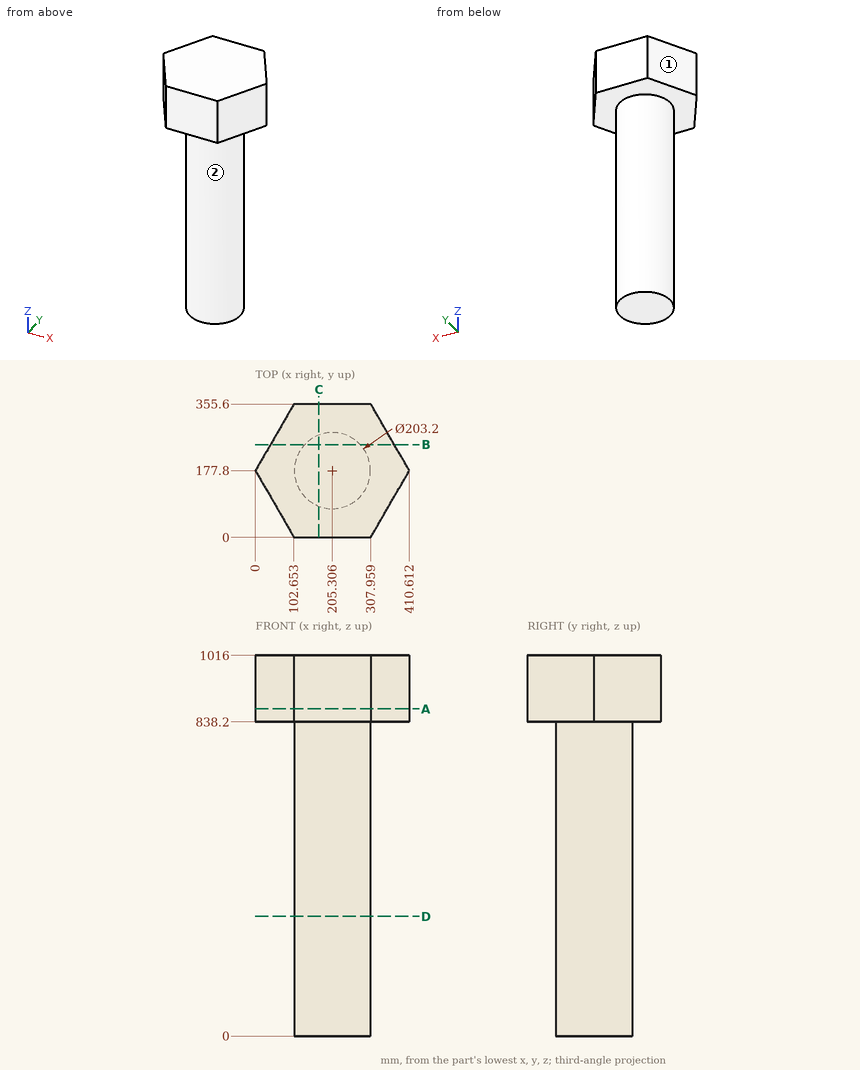
Drawing for the job (mm, zero at the part's lowest x, y, z). A direction names the side the tool comes from. Give positions to 0.01 mm unless a question says otherwise; leave off trailing zeros. Order: outer loops, then holes, each group sorted by start corner. A loop starts at its lowest first (then second) coordinate and runs counter-clockwise, first axis right, second up. Notation, with made-up numbers: (30, -30.75) -> (42, -30.75) arc R30 ccw to (42, 5.25) -> close; hole circle Ø10 at (69.5, 70.25). An arc over 180 degrees is marked (long way). Use one line per item in the form item = value.
(1) Saw through at A-A (z = 873). Write the cut outline in (x, y).
Solution:
outline = (0, 177.8) -> (102.65, 0) -> (307.96, 0) -> (410.61, 177.8) -> (307.96, 355.6) -> (102.65, 355.6) -> close
(2) Flat gauge pins, fed straight in: P1, Ø5, axis at x = 135.5, z = 650, coming from the +Y side; P2, Ø2, axis at y = 155, z = 817.5, coming from the -X side; P3, Ø5, axis at x = 112, y = 270.5, coming from the -Z side. Where does each tip first touch, or does it go through?
Solution:
P1 = 253.91
P2 = 106.07
P3 = 838.2
(3) Saw through at D-D (z = 319.5). Write the cut outline in (x, y) (1 decimal).
Solution:
outline = circle Ø203.2 at (205.3, 177.8)
(4) Saw through at C-C (x = 169.5). Write the cut outline in (y, z), then the cut area to 3 significant figures.
Solution:
outline = (0, 838.2) -> (82.72, 838.2) -> (82.72, 0) -> (272.88, 0) -> (272.88, 838.2) -> (355.6, 838.2) -> (355.6, 1016) -> (0, 1016) -> close
area = 223,000 mm²
(5) Drill centre lines: line 1 (Z direction, x = 294, y = 87); line 2 (X direction, y = 177, z = 565); line 3 (Y direction, x = 204.5, z = 168.5). Where is each one in solid material? Low to high. Write a range as from..to.
Solution:
line_1 = 838.2..1016
line_2 = 103.71..306.9
line_3 = 76.2..279.4
(6) Tool access for the marked faces 1 and 2: list every direction of +Z, -Z, +X, -X, +Y, -Y with a clear straight run to the whole face (end or side of a thin tool).
Solution:
face_1 = +Z, -Z, -X, +Y
face_2 = -Z
(7) Saw through at B-B (y = 247.5). Write the cut outline in (x, z), then the cut area to 3 significant figures.
Solution:
outline = (40.24, 838.2) -> (131.38, 838.2) -> (131.38, 0) -> (279.23, 0) -> (279.23, 838.2) -> (370.37, 838.2) -> (370.37, 1016) -> (40.24, 1016) -> close
area = 183,000 mm²
